For this review, take the finished solid that the model builds, in its own axes (mm). Face numbers are marked on the shaded views. A direction names the side the tool comes from. Coordinates: 2 decimals unless noted, no trailing zeros. Write each loop counter-clockwise with the first axis right and the second up, starting at its lowest first coordinate (ties: lowest second). Pieces come first, ordered by that corner, then holes. Notation, with made-up numbers: M 28,26.5 L 71,26.5 A35 ccw 71,65.5 Z; hole C 19,20.5 d4. An arc over 180 degrees is marked long. Return JSON: item names as keys, results as strings.
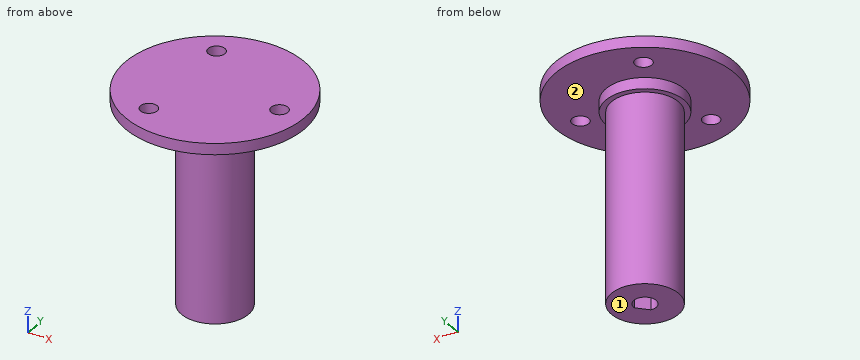
Autodesk Inventor part; units mm, degrees
ref_plane "YZ Plane" through (0, 0, 0) normal (1, 0, 0) x (0, 1, 0)
ref_plane "XZ Plane" through (0, 0, 0) normal (0, 1, 0) x (-1, 0, 0)
ref_plane "XY Plane" through (0, 0, 0) normal (0, 0, 1) x (1, 0, 0)
sketch "Skizze1" plane through (0, 0, 0) normal (0, 0, 1) x (1, 0, 0)
  circle A0 centre (0, 0) radius 16
  dimension "d0" = 32
extrude "Befestigungsfläche" add sketch "Skizze1" along normal blind 2
sketch "Skizze2" plane through (0, 0, 0) normal (0, 0, -1) x (-1, 0, 0)
  circle A0 centre (0, 0) radius 7
  dimension "d4" = 14
extrude "Mittelfläche" add sketch "Skizze2" along normal blind 2
sketch "Skizze3" plane through (0, 0, -2) normal (0, 0, -1) x (-1, 0, 0)
  circle A0 centre (0, 0) radius 6
  dimension "d7" = 12
extrude "Hauptkörper" add sketch "Skizze3" along normal blind 34
sketch "Skizze4" plane through (0, 0, -36) normal (0, 0, -1) x (-1, 0, 0)
  arc A0 (-0.1762, -1.9922) -> (-1.9922, -0.1762) centre (0, 0) ccw
  line L0 (-1.9922, -0.1762) -> (-0.1762, -1.9922)
  dimension "d10" = 4
extrude "Motorschaft (negativ)" cut sketch "Skizze4" against normal blind 10
sketch "Skizze6" plane through (0, 0, 2) normal (0, 0, 1) x (1, 0, 0)
  circle A0 centre (0, 0) radius 7
  line L0 (0, 0) -> (11.5, 0) construction
  line L1 (0, 0) -> (11.5, 0) construction
  circle A1 centre (11.5, 0) radius 1.5
  circle A2 centre (-5.75, 9.9593) radius 1.5
  circle A3 centre (-5.75, -9.9593) radius 1.5
  line L2 (0, 0) -> (11.5, 0)
  line L3 (0, 0) -> (-5.75, -9.9593)
  line L4 (0, 0) -> (11.5, 0) construction
  line L5 (0, 0) -> (-5.75, 9.9593)
  line L6 (0, 0) -> (11.5, 0) construction
  dimension "d14" = 14
  dimension "d21" = 3
  dimension "d22" = 3
  dimension "d23" = 3
  dimension "d26" = 11.5
  dimension "d27" = 11.5
  dimension "d28" = 120
  dimension "d29" = 11.5
  dimension "d30" = 120
extrude "Löcher" cut sketch "Skizze6" against normal blind 2 contours A3 | A2 | A1
properties part number "Motorbefestigung"
1. We need section B-B (z = -32.5). State the section outline as (x, y) points.
Checks:
{"outline": "C 0,0 d12; hole M 0.18,-1.99 L 1.99,-0.18 A2 ccw long Z"}
2. We need section A-A (x = 11). State the section outline as (y, z) points, plus the area to 3 significant figures.
Checks:
{"outline": "M -11.62,0 L -1.41,0 L -1.41,2 L -11.62,2 Z; M 1.41,0 L 11.62,0 L 11.62,2 L 1.41,2 Z", "area": "40.8 mm2"}
3. We need section D-D (z = -8.5). State the section outline as (x, y) points.
Checks:
{"outline": "C 0,0 d12"}
4. For the marked faces 1 and 2, list the 3-axis set-ups (+Z, -Z, +X, -X, +Y, -Y) from which the entire face can be reached by the end or side of a thin tool; tool diameter is ignored.
Checks:
{"face 1": "-Z, +X, -X, +Y, -Y", "face 2": "-Z"}
5. Wall thickness on L1, parallel to Y at x = -5.75, z = 0.6; L2, parallel to Z at x = -8, y = 5.5; L3, parallel to Y at x = -5, z = 1: over which ranges is each line inside the solid? List them lowest first. Write a range as from..to.
Checks:
{"L1": "-14.93..-11.46, -8.46..8.46, 11.46..14.93", "L2": "0..2", "L3": "-15.2..-11.26, -8.66..8.66, 11.26..15.2"}
6. Clearance check with flat-ended pins moving along their axes: pin 1 Ø1.5 at (y, z) = (1.5, -13) entering from -X; pin 2 Ø1 at (y, z) = (5, -8) entering from +X; pin 3 Ø12 at (x, z) = (-2, -16.5) entering from -Y; pin 4 Ø4 at (x, y) = (11.5, 0) entering from +Z. State where each tip first meets the part, or that it passes through.
Checks:
{"pin 1": "x = -5.95", "pin 2": "x = 3.97", "pin 3": "y = -6", "pin 4": "z = 2"}
7. We need section C-C (y = 5.5). State the section outline as (x, z) points.
Checks:
{"outline": "M -15.02,0 L -4.33,0 L -4.33,-2 L -2.4,-2 L -2.4,-36 L 2.4,-36 L 2.4,-2 L 4.33,-2 L 4.33,0 L 15.02,0 L 15.02,2 L -15.02,2 Z"}
